Geometry: final body of the model. Coordinates: model frame, mm. A direction names the side the tool comes from. Give positions to 0.01 mm unless a question says otherwise; leave off trailing zeros. Write each loop counter-clockwise with the first axis right and the second up, starting at its lowest first coordinate (ties: lowest second). Pieces come first, ordered by that corner, then holes.
```python
from build123d import *

# Parameters (mm, degrees)
BOX006_W               = 25
BOX006_H               = 40
BOX006_DEPTH           = 4
BOX006_ROLL_ANGLE      = 45
BOX006_PLACEMENT_ANGLE = 90
BOX005_W               = 25
BOX005_H               = 40
BOX005_DEPTH           = 4
BOX005_ROLL_ANGLE      = 45
BOX005_PLACEMENT_ANGLE = 90
CYLINDER014_R          = 4
CYLINDER014_DEPTH      = 20
CYLINDER015_R          = 4
CYLINDER015_DEPTH      = 20
CYLINDER016_R          = 4
CYLINDER016_DEPTH      = 20
CYLINDER011_R          = 2
CYLINDER011_DEPTH      = 30
CYLINDER012_R          = 2
CYLINDER012_DEPTH      = 30
CYLINDER013_R          = 2
CYLINDER013_DEPTH      = 30
CYLINDER009_R          = 4
CYLINDER009_DEPTH      = 10
CYLINDER010_R          = 4
CYLINDER010_DEPTH      = 10
CYLINDER008_R          = 4
CYLINDER008_DEPTH      = 10
BOX001_W               = 70
BOX001_H               = 20
BOX001_DEPTH           = 20
BOX_W                  = 91
BOX_H                  = 56
BOX_DEPTH              = 20
BOX002_W               = 10.5
BOX002_H               = 35
BOX002_DEPTH           = 17
CYLINDER006_R          = 3.65
CYLINDER006_DEPTH      = 10
BOX003_W               = 75
BOX003_H               = 150
BOX003_DEPTH           = 25
FILLET_R               = 5
FILLET001_R            = 5
FILLET002_R            = 5
FILLET003_R            = 5
FILLET004_R            = 5
FILLET005_R            = 5
CYLINDER003_R          = 8.75
CYLINDER003_DEPTH      = 40
CYLINDER002_R          = 2
CYLINDER002_DEPTH      = 10
ARRAY_COUNT            = 3
CYLINDER001_R          = 2.25
CYLINDER001_DEPTH      = 5
CYLINDER_R             = 35
CYLINDER_DEPTH         = 18
CYLINDER004_R          = 35
CYLINDER004_DEPTH      = 25
CYLINDER005_R          = 8.75
CYLINDER005_DEPTH      = 40
CYLINDER007_R          = 10.75
CYLINDER007_DEPTH      = 40
BOX004_W               = 99
BOX004_H               = 150
BOX004_DEPTH           = 32


with BuildPart() as slot2:
    # Box006 → Box006 (new body)
    with BuildSketch(Plane.XY):
        with Locations((12.5, 20)):
            Rectangle(BOX006_W, BOX006_H)
    extrude(amount=BOX006_DEPTH)


with BuildPart() as slot2_1:
    # Box006 roll: moved
    add(slot2.part.rotate(Axis((0, 0, 0), (1, 0, 0)), BOX006_ROLL_ANGLE))


with BuildPart() as slot2_2:
    # Box006 placement: moved
    add(slot2_1.part.moved(Location((-37.422836, -44, -17.67767))).rotate(Axis((-37.422836, -44, -17.67767), (0, 0, 1)), BOX006_PLACEMENT_ANGLE))


with BuildPart() as part_mirroring:
    # Part__Mirroring: instance of Slot2
    add(slot2_2.part.mirror(Plane(origin=(0, 0, 0), x_dir=(0, -1, 0), z_dir=(1, 0, 0))))


with BuildPart() as part_mirroring_1:
    # Part__Mirroring placement: moved
    add(part_mirroring.part.moved(Location((0, -7, 0))))


with BuildPart() as strapslots:
    # Box005 → Box005 (new body)
    with BuildSketch(Plane.XY):
        with Locations((12.5, 20)):
            Rectangle(BOX005_W, BOX005_H)
    extrude(amount=BOX005_DEPTH)


with BuildPart() as strapslots_1:
    # Box005 roll: moved
    add(strapslots.part.rotate(Axis((0, 0, 0), (1, 0, 0)), BOX005_ROLL_ANGLE))


with BuildPart() as strapslots_2:
    # Box005 placement: moved
    add(strapslots_1.part.moved(Location((-37.422836, -51, -17.67767))).rotate(Axis((-37.422836, -51, -17.67767), (0, 0, 1)), BOX005_PLACEMENT_ANGLE))

    # Fusion011: union Part__Mirroring
    add(part_mirroring_1.part)


with BuildPart() as cylinder009:
    # Cylinder014 → Cylinder014 (new body)
    with BuildSketch(Plane(origin=(37.5, -21, 10), x_dir=(1, 0, 0), z_dir=(0, 0, 1))):
        Circle(CYLINDER014_R)
    extrude(amount=CYLINDER014_DEPTH)


with BuildPart() as cylinder010:
    # Cylinder015 → Cylinder015 (new body)
    with BuildSketch(Plane(origin=(37.5, 23, 10), x_dir=(1, 0, 0), z_dir=(0, 0, 1))):
        Circle(CYLINDER015_R)
    extrude(amount=CYLINDER015_DEPTH)


with BuildPart() as mounting002:
    # Cylinder016 → Cylinder016 (new body)
    with BuildSketch(Plane(origin=(-41.5, -1, 10), x_dir=(1, 0, 0), z_dir=(0, 0, 1))):
        Circle(CYLINDER016_R)
    extrude(amount=CYLINDER016_DEPTH)

    # Fusion008: union Cylinder009, Cylinder010
    add(cylinder009.part)
    add(cylinder010.part)


with BuildPart() as mounting002_1:
    # Fusion008 placement: moved
    add(mounting002.part.moved(Location((0, 0, -30))))


with BuildPart() as cylinder006:
    # Cylinder011 → Cylinder011 (new body)
    with BuildSketch(Plane(origin=(37.5, -21, 10), x_dir=(1, 0, 0), z_dir=(0, 0, 1))):
        Circle(CYLINDER011_R)
    extrude(amount=CYLINDER011_DEPTH)


with BuildPart() as cylinder007:
    # Cylinder012 → Cylinder012 (new body)
    with BuildSketch(Plane(origin=(37.5, 23, 10), x_dir=(1, 0, 0), z_dir=(0, 0, 1))):
        Circle(CYLINDER012_R)
    extrude(amount=CYLINDER012_DEPTH)


with BuildPart() as bottommounting:
    # Cylinder013 → Cylinder013 (new body)
    with BuildSketch(Plane(origin=(-41.5, -1, 10), x_dir=(1, 0, 0), z_dir=(0, 0, 1))):
        Circle(CYLINDER013_R)
    extrude(amount=CYLINDER013_DEPTH)

    # Fusion007: union Cylinder006, Cylinder007
    add(cylinder006.part)
    add(cylinder007.part)


with BuildPart() as bottommounting_1:
    # Fusion007 placement: moved
    add(bottommounting.part.moved(Location((0, 0, -30))))

    # Fusion009: union Mounting002
    add(mounting002_1.part)


with BuildPart() as cylinder004:
    # Cylinder009 → Cylinder009 (new body)
    with BuildSketch(Plane(origin=(37.5, -21, 10), x_dir=(1, 0, 0), z_dir=(0, 0, 1))):
        Circle(CYLINDER009_R)
    extrude(amount=CYLINDER009_DEPTH)


with BuildPart() as cylinder005:
    # Cylinder010 → Cylinder010 (new body)
    with BuildSketch(Plane(origin=(37.5, 23, 10), x_dir=(1, 0, 0), z_dir=(0, 0, 1))):
        Circle(CYLINDER010_R)
    extrude(amount=CYLINDER010_DEPTH)


with BuildPart() as combinedmounting:
    # Cylinder008 → Cylinder008 (new body)
    with BuildSketch(Plane(origin=(-41.5, -1, 10), x_dir=(1, 0, 0), z_dir=(0, 0, 1))):
        Circle(CYLINDER008_R)
    extrude(amount=CYLINDER008_DEPTH)

    # Fusion006: union Cylinder004, Cylinder005
    add(cylinder004.part)
    add(cylinder005.part)

    # Fusion010: union BottomMounting
    add(bottommounting_1.part)


with BuildPart() as wiringpocket:
    # Box001 → Box001 (new body)
    with BuildSketch(Plane(origin=(-35, -53, 0), x_dir=(1, 0, 0), z_dir=(0, 0, 1))):
        with Locations((35, 10)):
            Rectangle(BOX001_W, BOX001_H)
    extrude(amount=BOX001_DEPTH)


with BuildPart() as electronicspocket:
    # Box → Box (new body)
    with BuildSketch(Plane(origin=(-45.5, -106, 0), x_dir=(1, 0, 0), z_dir=(0, 0, 1))):
        with Locations((45.5, 28)):
            Rectangle(BOX_W, BOX_H)
    extrude(amount=BOX_DEPTH)

    # Fusion: union WiringPocket
    add(wiringpocket.part)


with BuildPart() as electronicspocket_1:
    # Fusion placement: moved
    add(electronicspocket.part.moved(Location((0, 5, 0))))


with BuildPart() as potentiometer:
    # Box002 → Box002 (new body)
    with BuildSketch(Plane(origin=(-30, 18, 5.5), x_dir=(1, 0, 0), z_dir=(0, 0, 1))):
        with Locations((5.25, 17.5)):
            Rectangle(BOX002_W, BOX002_H)
    extrude(amount=BOX002_DEPTH)


with BuildPart() as potpocket:
    # Cylinder006 → Cylinder006 (new body)
    with BuildSketch(Plane(origin=(-24.75, 60.5, 11), x_dir=(1, 0, 0), z_dir=(0, -1, 0))):
        Circle(CYLINDER006_R)
    extrude(amount=CYLINDER006_DEPTH)

    # Fusion001: union Potentiometer
    add(potentiometer.part)


with BuildPart() as potpocket_1:
    # Fusion001 placement: moved
    add(potpocket.part.moved(Location((-3.5, -10, -2.5))))


with BuildPart() as batterypocket:
    # Box003 → Box003 (new body)
    with BuildSketch(Plane(origin=(-37.5, -101, -29), x_dir=(1, 0, 0), z_dir=(0, 0, 1))):
        with Locations((37.5, 75)):
            Rectangle(BOX003_W, BOX003_H)
    extrude(amount=BOX003_DEPTH)

    # Fillet
    fillet_edges = [batterypocket.edges().sort_by_distance(p)[0] for p in [
        (-37.5, -26, -4),
    ]]
    fillet(fillet_edges, radius=FILLET_R)

    # Fillet001
    fillet001_edges = [batterypocket.edges().sort_by_distance(p)[0] for p in [
        (-37.5, -26, -29),
    ]]
    fillet(fillet001_edges, radius=FILLET001_R)

    # Fillet002
    fillet002_edges = [batterypocket.edges().sort_by_distance(p)[0] for p in [
        (37.5, -26, -29),
    ]]
    fillet(fillet002_edges, radius=FILLET002_R)

    # Fillet003
    fillet003_edges = [batterypocket.edges().sort_by_distance(p)[0] for p in [
        (37.5, -26, -4),
    ]]
    fillet(fillet003_edges, radius=FILLET003_R)

    # Fillet004
    fillet004_edges = [batterypocket.edges().sort_by_distance(p)[0] for p in [
        (0, 49, -29),
    ]]
    fillet(fillet004_edges, radius=FILLET004_R)

    # Fillet005
    fillet005_edges = [batterypocket.edges().sort_by_distance(p)[0] for p in [
        (37.5, -101, -16.5),
        (0, -101, -4),
        (0, -101, -29),
        (-37.5, -101, -16.5),
    ]]
    fillet(fillet005_edges, radius=FILLET005_R)


with BuildPart() as obj1:
    # Cone → Cone (revolve)
    with BuildSketch(Plane(origin=(0, 0, 22.5), x_dir=(1, 0, 0), z_dir=(0, -1, 0))):
        Polygon((0, 0), (27.25, 0), (27.15, 13), (0, 13), align=None)
    revolve(axis=Axis((0, 0, 22.5), (0, 0, 1)))


with BuildPart() as bloweroutlet:
    # Cylinder003 → Cylinder003 (new body)
    with BuildSketch(Plane(origin=(20, 36.3, 13.5), x_dir=(1, 0, 0), z_dir=(0, -1, 0))):
        Circle(CYLINDER003_R)
    extrude(amount=CYLINDER003_DEPTH)


with BuildPart() as blowerfeet:
    # Cylinder002 → Cylinder002 (new body)
    with BuildSketch(Plane(origin=(0, -28.4, 0), x_dir=(1, 0, 0), z_dir=(0, 0, 1))):
        Circle(CYLINDER002_R)
    extrude(amount=CYLINDER002_DEPTH)

    # Array: BlowerFeet ×3 about axis
    array_axis = Axis((0, 0, 0), (0, 0, 1))


with BuildPart() as blowerfeet_1:
    add(blowerfeet.part)
    for i in range(1, ARRAY_COUNT):
        add(blowerfeet.part.rotate(array_axis, i * 360 / ARRAY_COUNT))


with BuildPart() as blowerendbearing:
    # Cylinder001 → Cylinder001 (new body)
    with BuildSketch(Plane.XY.offset(1)):
        Circle(CYLINDER001_R)
    extrude(amount=CYLINDER001_DEPTH)


with BuildPart() as blowerbody:
    # Cylinder → Cylinder (new body)
    with BuildSketch(Plane.XY.offset(4.5)):
        Circle(CYLINDER_R)
    extrude(amount=CYLINDER_DEPTH)


with BuildPart() as blowerpocket:
    # Cylinder004 → Cylinder004 (new body)
    with BuildSketch(Plane.XY):
        Circle(CYLINDER004_R)
    extrude(amount=CYLINDER004_DEPTH)

    # Fusion003: union obj1, BlowerOutlet, BlowerFeet, BlowerEndbearing, BlowerBody
    add(obj1.part)
    add(bloweroutlet.part)
    add(blowerfeet_1.part)
    add(blowerendbearing.part)
    add(blowerbody.part)


with BuildPart() as combinedpocket:
    # Cylinder005 → Cylinder005 (new body)
    with BuildSketch(Plane(origin=(20, 65.3, 13.5), x_dir=(1, 0, 0), z_dir=(0, -1, 0))):
        Circle(CYLINDER005_R)
    extrude(amount=CYLINDER005_DEPTH)

    # Fusion004: union ElectronicsPocket, PotPocket, BatteryPocket, BlowerPocket
    add(electronicspocket_1.part)
    add(potpocket_1.part)
    add(batterypocket.part)
    add(blowerpocket.part)


with BuildPart() as housingoutlet:
    # Cylinder007 → Cylinder007 (new body)
    with BuildSketch(Plane(origin=(20, 59.3, 13.5), x_dir=(1, 0, 0), z_dir=(0, -1, 0))):
        Circle(CYLINDER007_R)
    extrude(amount=CYLINDER007_DEPTH)


with BuildPart() as housingblock:
    # Box004 → Box004 (new body)
    with BuildSketch(Plane(origin=(-49.5, -105, -12), x_dir=(1, 0, 0), z_dir=(0, 0, 1))):
        with Locations((49.5, 75)):
            Rectangle(BOX004_W, BOX004_H)
    extrude(amount=BOX004_DEPTH)


with BuildPart() as obj2:
    # Cone001 → Cone001 (revolve)
    with BuildSketch(Plane(origin=(20, 65.3, 13.5), x_dir=(-1, 0, 0), z_dir=(0, 0, 1))):
        Polygon((0, 0), (10.92, 0), (11.19, 21), (0, 21), align=None)
    revolve(axis=Axis((20, 65.3, 13.5), (0, -1, 0)))

    # Fusion005: union HousingOutlet, HousingBlock
    add(housingoutlet.part)
    add(housingblock.part)

    # Cut: cut CombinedPocket
    add(combinedpocket.part, mode=Mode.SUBTRACT)

    # Cut001: cut CombinedMounting
    add(combinedmounting.part, mode=Mode.SUBTRACT)

    # Cut002: cut StrapSlots
    add(strapslots_2.part, mode=Mode.SUBTRACT)


solid = obj2.part
```
Item 1: Pull-direction query (Z, two-part tool) for faces 1 (the face through (-45, -51, -7)), 2 (the face through (39, 21, 0)), 3 (the face through (-44.7, -3.4, 14.9)); classes: +Z half, -Z half, draft (parallel to the pull), parting line (faces both ways), or undercut.
Found:
face 1: undercut
face 2: -Z half
face 3: draft
Item 2: Section C-C, the plane z = 17.5. State how many separate pieces and enclosed holes the cut face has, plus the area to 3 significant figures.
Found:
separate pieces: 1
enclosed holes: 3
area: 4,360 mm2
Item 3: Section B-B, the plane x = 0. Return the cut outline in (y, z), plus the area to 3 significant figures.
Found:
outline: (-105, -12) - (-101, -12) - (-101, -9) arc R5 cw to (-96, -4) - (44, -4) arc R5 cw to (45, -4.1) - (45, 20) - (35, 20) - (35, 0) - (-101, 0) - (-101, 20) - (-105, 20) - close
area: 917 mm2
Item 4: Pin query (flat end, axial travel): pin 1 Ø6.5 at (x, y) = (37.5, -21) entering from +Z; pin 2 Ø2.5 at (x, y) = (-40, -1.5) entering from -Z; pin 3 Ø6.5 at (x, z) = (-28.25, 8.5) entering from +Y. Return the tip coordinate at first contact, or that it passes through.
Found:
pin 1: stops at z = 10
pin 2: stops at z = 0
pin 3: stops at y = -15.26
Item 5: Line query: L1, parallel to Y at x = 37.5, z = -4.25; L2, parallel to Y at x = 37.5, z = 18.25; L3, parallel to Y at x = 37.5, z = 3. Output: solid intervals per line, ascending.
Found:
L1: y = -105 to -25, -17 to 19, 27 to 45
L2: y = -105 to -101, -45 to -25, -17 to 19, 27 to 45
L3: y = -105 to -101, -45 to -23, -19 to 21, 25 to 45
Item 6: Reachability of faces 4 (the face through (34.55, -18.3, 14.93)), 5 (the face through (-40, -3, 0)), 6 (the face through (45, -26, -7)) from +Z, -Z, +X, -X, +Y, -Y: full face, straight path, thin tool, end or side. Return the list, or none.
Found:
face 4: +Z
face 5: -Z
face 6: none
